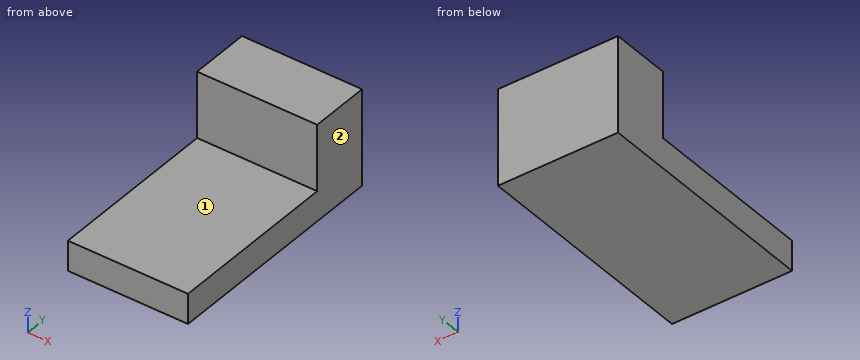
from build123d import *

# Parameters (mm, degrees)
SKETCH1_W           = 12.7
SKETCH1_H           = 49.300000012
BOSS_EXTRUDE1_DEPTH = 6.35
SKETCH3_W           = 6.35
SKETCH3_H           = 49.300000012
BOSS_EXTRUDE3_DEPTH = 12.7
SKETCH2_W           = 25.4
SKETCH2_H           = 12.7
BOSS_EXTRUDE2_DEPTH = 13.97


with BuildPart() as part:
    # Sketch1 → Boss-Extrude1 (new body)
    with BuildSketch(Plane.XY):
        with Locations((-9.26915446, 7.290553641)):
            Rectangle(SKETCH1_W, SKETCH1_H)
    extrude(amount=BOSS_EXTRUDE1_DEPTH)

    # Sketch3 → Boss-Extrude3 (add)
    with BuildSketch(Plane.ZY.offset(15.61915446)):
        with Locations((3.175, 7.290553641)):
            Rectangle(SKETCH3_W, SKETCH3_H)
    extrude(amount=BOSS_EXTRUDE3_DEPTH)

    # Sketch2 → Boss-Extrude2 (add)
    with BuildSketch(Plane.XY.offset(6.35)):
        with Locations((-15.61915446, 25.590553647)):
            Rectangle(SKETCH2_W, SKETCH2_H)
    extrude(amount=BOSS_EXTRUDE2_DEPTH)


solid = part.part
Geometry: final body of the model. Coordinates: model frame, mm. Face numbers are marked on the shaded views. A direction names the side the tool comes from. Coordinates: 2 decimals unless noted, no trailing zeros. Loops run counter-clockwise (first coordinate to the right, second up) from the corner with the lowest first, then second, coordinate; pieces in that order, holes last. Notation, with made-up numbers: M 59,-30.75 L 92,-30.75 A13 cw 92,-9.75 Z; hole C 14,30.25 d11. An arc over 180 degrees is marked long. One line per item, written item: value. Start each with the question number.
1) Cut plane B-B (y = 12.5). Return loops of the section in (x, z).
2) Cut plane A-A (x = -25.25). Return loops of the section in (y, z), then the cut area to 3 significant figures.
3) Reachability of the marked faces 1 and 2 from +Z, -Z, +X, -X, +Y, -Y: full face, straight path, thin tool, end or side. Return the list, or none.
4) Pin query (flat end, axial travel): P1, Ø7.5, axis at x = -15, y = -4.5, coming from the +Z side; P2, Ø12, axis at y = 8.5, z = 15.5, coming from the +X side; P3, Ø7, axis at x = -13, z = 14.5, coming from the -Y side. Return the tip coordinate at first contact, or that it passes through.
5) Material intervals for L1, parallel to Z at x = -17, y = 0; L2, parallel to Y at x = -10.25, z = 18.25, sorted ascending. Write a range as from..to.
Evaluation:
1. outline: M -28.32,0 L -2.92,0 L -2.92,6.35 L -28.32,6.35 Z
2. outline: M -17.36,0 L 31.94,0 L 31.94,20.32 L 19.24,20.32 L 19.24,6.35 L -17.36,6.35 Z
2. area: 490 mm^2
3. face 1: +Z, +X, -X, -Y
3. face 2: +Z, -Z, +X, +Y, -Y
4. P1: z = 6.35
4. P2: through
4. P3: y = 19.24
5. L1: 0..6.35
5. L2: 19.24..31.94
